Could you check a few things on this model? Use its own coordinates, in mm. Face numbers are marked on the shaded views. Coordinates: 2 decimals unless noted, no trailing zeros. Loops run counter-clockwise (first coordinate to the right, second up) from the corner with the lowest first, then second, coordinate; pieces in that order, holes last. Notation, with made-up numbers: M 33,19 L 62,19 A20 cw 62,54 Z; hole C 74.5,-5.75 d3. An arc over 180 degrees is marked long. Use one line per item in the form item = value. Start each with the question number.
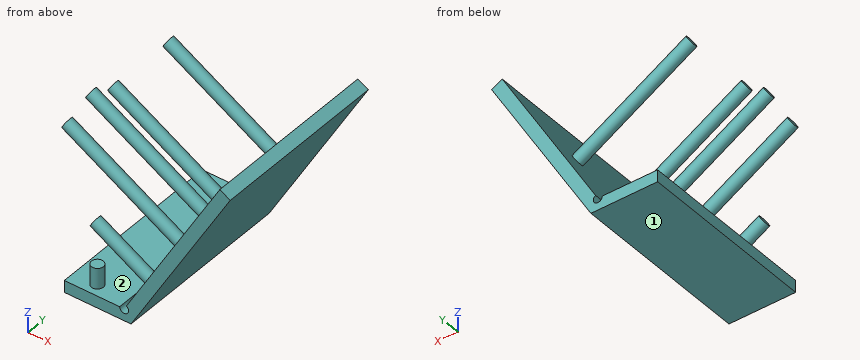
```python
from build123d import *

# Parameters (mm, degrees)
F1_DEPTH = 190.5
F2_R     = 6.35
F4_DEPTH = 21.9964
F3_R     = 6.35
F5_DEPTH = 68.1482
F6_DEPTH = 139.7


with BuildPart() as f1:
    # F0 (on Front) → F1 (new body)
    with BuildSketch(Plane.XZ):
        with BuildLine():
            Line((58.745752, 0), (0, 0))
            Line((0, 0), (0, -12.7))
            Line((0, -12.7), (70.8406, -12.7))
            Line((70.8406, -12.7), (176.1109, 169.633508))
            Line((176.1109, 169.633508), (165.112377, 175.983508))
            Line((165.112377, 175.983508), (65.889502, 4.124446))
            ThreePointArc((65.889502, 4.124446), (65.889502, -4.124446), (58.745752, 0))
        make_face()
    extrude(amount=F1_DEPTH)

    # F2 (on face) → F4 (join)
    with BuildSketch(Plane.XY):
        with Locations((25.4, -177.8)):
            Circle(F2_R)
    extrude(amount=F4_DEPTH)

    # F3 (on face) → F5 (join)
    with BuildSketch(Plane(origin=(47.631189, 0, -27.49988), x_dir=(0, -1, 0), z_dir=(-0.866025, 0, 0.5))):
        with Locations((177.8, 69.862377)):
            Circle(F3_R)
    extrude(amount=F5_DEPTH)

    # F3 (on face) → F6 (join)
    with BuildSketch(Plane(origin=(47.631189, 0, -27.49988), x_dir=(0, -1, 0), z_dir=(-0.866025, 0, 0.5))):
        with Locations((177.8, 133.362377)):
            Circle(F3_R)
        with Locations((114.3, 133.362377)):
            Circle(F3_R)
        with Locations((38.1, 133.362377)):
            Circle(F3_R)
        with Locations((177.8, 184.162377)):
            Circle(F3_R)
    extrude(amount=F6_DEPTH)


solid = f1.part
```
Item 1: Thinking about a two-plate mould opening in Z: for the marked faces 1 and 2, which applies, pulls with the +Z half, pulls with the -Z half, needs draft (parallel to the pull), parting line crosses it, or undercut?
Item 2: I'm going to push flat-ended pins straight in: P1, Ø1.5, axis at y = -137, z = 50.5, coming from the -X side; P2, Ø12, axis at x = 53, z = 112.5, coming from the -Y side; P3, Ø8.5, axis at x = 63.51, z = 0, coming from the -Y side; P4, Ø1, axis at x = 46.5, y = -25, coming from the +Z side. Where does each tip first touch, or does it pass through?
Item 3: Please list where these lines run through material, in increasing order: line 1 along Z through (x, y) = (146, -125); line 2 along Z through (x, y) = (2, -39); line 3 along Z through (x, y) = (29, -175).
Item 4: I want a section at B-B (x = 109). Count the separate pieces of the cut face and the enclosed holes in it, plus the area to 3 significant figures.
Item 5: I want a section at A-A (y = -124). Write out the boundary of the cut face in (x, z) (1 decimal).
Worked answers:
q1.face_1 = pulls with the -Z half
q1.face_2 = undercut
q2.P1 = 92.23
q2.P2 = -183.14
q2.P3 = through
q2.P4 = 0
q3.line_1 = 117.48 to 142.88
q3.line_2 = -12.7 to 0, 145.58 to 160.1
q3.line_3 = -12.7 to 22, 57.35 to 70.51, 130.67 to 143.83, 189.33 to 202.49
q4.separate_pieces = 5
q4.enclosed_holes = 0
q4.area = 5,420 mm²
q5.outline = M 0,-12.7 L 70.8,-12.7 L 176.1,169.6 L 165.1,176 L 65.9,4.1 A4.8 cw long 58.7,0 L 0,0 Z
